Verification items for the finished model (mm, model axes). Face numbers are marked on the shaded views. A direction names the side the tool comes from. Give positions to 0.01 mm unless a question says otherwise; leave off trailing zeros. Loops run counter-clockwise (first coordinate to the right, second up) from the corner with the lowest first, then second, coordinate; pieces in that order, holes last. Notation, with made-up numbers: (-22.75, -20.5) - (-18.75, -20.5) arc R29 ccw to (-18.75, 15.5) - close; hole circle Ø2 at (-35.5, 32). An arc over 180 degrees is marked (long way). One line per question, with ' | ' between items. Start each with the question number.
1. Section check C-C, the plane z = -3.5. Enter the section's corners in (x, y).
2. Section check D-D, the plane x = 6.5. Enter the section's corners in (y, z).
3. Mould release check, pull along Z, two halves, no side actions. Record for the marked faces 1, 2 and 3: +Z half, -Z half, draft (parallel to the pull), parting line (faces both ways), or undercut.
4. Section check B-B, the plane y = 1.25. Enter the section's corners in (x, z).
5. Section check A-A, the plane z = 0. Enter the section's corners in (x, y), then the cut area to 3 significant figures.
6. Tool access check on the marked faces 4, 5, 6 and 7. Record the directions out of +Z, -Z, +X, -X, +Y, -Y that give a thin tool (end or side, any length) a straight path to the whole face; none if there is none.
7. Depth check by flat-ended pin: pin 1 Ø3 at (x, z) = (6, 0) entering from -Y (3 decimals); pin 2 Ø0.6 at (x, y) = (5, 1) entering from -Z; pin 3 Ø3 at (x, z) = (6.5, 1.5) entering from +Y; pin 4 Ø1.5 at (y, z) = (6.5, 2) entering from +X. Enter the tip coordinate at first touch or a pass-through.
8. Thickness scan on line 1 along X through (y, z) = (1.6, 0); line 2 along Y through (x, z) = (1.5, -0.25); line 3 along X through (y, z) = (0.5, -0.5). Record the ranges inside material, lowest first. Write a range as from..to.
from build123d import *

# Parameters (mm, degrees)
SKETCH_1_R            = 1.6
EXTRUDE_330_DEPTH     = 2
SKETCH_2_W            = 5
SKETCH_2_H            = 10
EXTRUDE_541_DEPTH     = 12.2
SKETCH_3_W            = 5
SKETCH_3_H            = 3
CUT_EXTRUDE_754_DEPTH = 7.5


with BuildPart() as part:
    # Эскиз1 → Extrude 330 (new body)
    with BuildSketch(Plane(origin=(0, 0, 0), x_dir=(1, 0, 0), z_dir=(0, 1, 0))):
        with BuildLine():
            Line((-6, 3), (6, 3))
            ThreePointArc((6, 3), (9, 0), (6, -3))
            Line((6, -3), (-6, -3))
            ThreePointArc((-6, -3), (-9, 0), (-6, 3))
        make_face()
        with Locations(Location((-6, 0, 0), (0, 0, 270))):
            Circle(SKETCH_1_R, mode=Mode.SUBTRACT)
        with Locations(Location((6, 0, 0), (0, 0, 270))):
            Circle(SKETCH_1_R, mode=Mode.SUBTRACT)
    extrude(amount=EXTRUDE_330_DEPTH)

    # Эскиз2 → Extrude 541 (add)
    with BuildSketch(Plane.XZ):
        with Locations((0, -2)):
            Rectangle(SKETCH_2_W, SKETCH_2_H)
    extrude(amount=-EXTRUDE_541_DEPTH)

    # Эскиз3 → Cut-Extrude 754 (cut)
    with BuildSketch(Plane(origin=(0, 0, -7), x_dir=(-1, 0, 0), z_dir=(0, 0, -1))):
        with Locations((0, 6.1)):
            Rectangle(SKETCH_3_W, SKETCH_3_H)
    extrude(amount=-CUT_EXTRUDE_754_DEPTH, mode=Mode.SUBTRACT)


solid = part.part
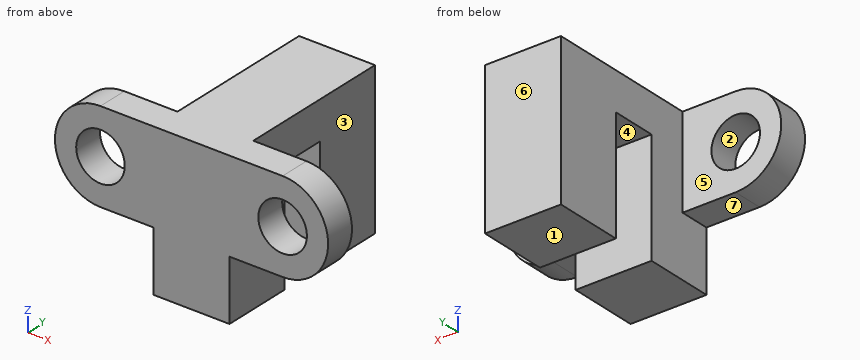
Results list:
1) outline: (-2.5, 0) - (2.5, 0) - (2.5, 4.6) - (-2.5, 4.6) - close; (-2.5, 7.6) - (2.5, 7.6) - (2.5, 12.2) - (-2.5, 12.2) - close
2) outline: (0, -2.96) - (2, -2.96) - (2, -1.52) - (0, -1.52) - close; (0, 1.52) - (2, 1.52) - (2, 2.96) - (0, 2.96) - close
3) face 1: -Z half | face 2: undercut | face 3: draft
4) outline: (-6, -3) - (-2.5, -3) - (-2.5, -7) - (2.5, -7) - (2.5, -3) - (6, -3) arc R3 ccw to (6, 3) - (-6, 3) arc R3 ccw to start; hole circle Ø3.2 at (-6, 0); hole circle Ø3.2 at (6, 0)
5) outline: (-9, 0) - (-7.6, 0) - (-7.6, 2) - (-9, 2) - close; (-4.4, 0) - (4.4, 0) - (4.4, 2) - (2.5, 2) - (2.5, 4.6) - (-2.5, 4.6) - (-2.5, 2) - (-4.4, 2) - close; (-2.5, 7.6) - (2.5, 7.6) - (2.5, 12.2) - (-2.5, 12.2) - close; (7.6, 0) - (9, 0) - (9, 2) - (7.6, 2) - close | area: 59.2 mm²
6) face 4: -Z, +X, -X | face 5: +Z, -Z, -X, +Y | face 6: +Z, -Z, +X, -X, +Y | face 7: -Z, -X, +Y, -Y
7) pin 1: through | pin 2: z = -3 | pin 3: y = 2 | pin 4: x = 2.5
8) line 1: -9..-7.6, -4.4..4.4, 7.6..9 | line 2: 0..4.6, 7.6..12.2 | line 3: -8.96..-7.52, -4.48..4.48, 7.52..8.96
